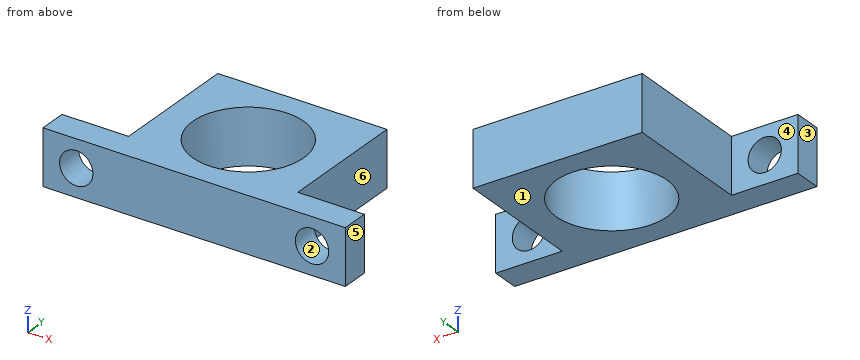
from build123d import *

# Parameters (mm, degrees)
SKETCH_1_R          = 10
EXTRUDE_1_DEPTH     = 10
SKETCH_2_R          = 3
CUT_EXTRUDE_1_DEPTH = 43.114991393


with BuildPart() as part:
    # 草图1 → 凸台-拉伸1 (new body)
    with BuildSketch(Plane.XY):
        Polygon((17.35, 7.3), (-13.15, 7.3), (-13.15, -16.2), (-25.15, -16.2), (-25.15, -21.2), (29.35, -21.2), (29.35, -16.2), (17.35, -16.2), align=None)
        with Locations((2.1, -6.95)):
            Circle(SKETCH_1_R, mode=Mode.SUBTRACT)
    extrude(amount=EXTRUDE_1_DEPTH)

    # 草图2 → 切除-拉伸1 (cut, through all)
    with BuildSketch(Plane(origin=(0, 7.3, 0), x_dir=(1, 0, 0), z_dir=(0, 1, 0))):
        with Locations(Location((-19.15, -5, 0), (0, 0, 180))):
            Circle(SKETCH_2_R)
        with Locations((23.35, -5)):
            Circle(SKETCH_2_R)
    extrude(amount=-CUT_EXTRUDE_1_DEPTH, mode=Mode.SUBTRACT)


solid = part.part
Design review of the part built by this model. Coordinates are the model's own, in mm. Face numbers are marked on the shaded views. A direction names the side the tool comes from. Coordinates: 2 decimals unless noted, no trailing zeros. Order: outer loops, then holes, each group sorted by start corner. A loop starts at its lowest first (then second) coordinate and runs counter-clockwise, first axis right, second up.
Item 1: Take a section at B-B, the plane x = -19.15. Write out the cut boundary in (y, z), then the cut area to 3 significant figures.
Item 2: For line 1 (X direction, y = -17.25, z = 4.75); line 2 (Z direction, x = 23.35, y = -19.7); line 3 (X direction, y = -19.75, z = 7.5), list the stretches that pass through material, from the lowest coordinate up.
Item 3: For pin 1 Ø3 at (y, z) = (-4, 3) entering from -X; pin 2 Ø6 at (y, z) = (-0.5, 3) entering from +X; pin 3 Ø3 at (x, z) = (-18.5, 6.5) entering from +Y, all flat-tipped, find the tip position at first contact; note any pin that passes through.
Item 4: Take a section at C-C, the plane y = -6.95. Write out the cut boundary in (x, z), then the cut area to 3 significant figures.
Item 5: Take a section at D-D, the plane z = 8.5. Write out the cut boundary in (x, y), then the cut area to 3 significant figures.
Item 6: For the marked faces 4, 5 and 6, list the 3-axis set-ups (+Z, -Z, +X, -X, +Y, -Y) from which the entire face can be reached by the end or side of a thin tool; tool diameter is ignored.
Item 7: The part is to be moulded in two halves that separate along X. For the marked faces 1, 2 and 3, say which applies: pulls with the +X half, pulls with the -X half, needs draft (parallel to the pull), parting line crosses it, or undercut.
Item 8: Take a section at A-A, the plane z = 5. Write out the cut boundary in (x, y).
The answers:
1. outline: (-21.2, 0) - (-16.2, 0) - (-16.2, 2) - (-21.2, 2) - close; (-21.2, 8) - (-16.2, 8) - (-16.2, 10) - (-21.2, 10) - close
1. area: 20.0 mm2
2. line 1: x = -25.15 to -22.14, -16.16 to 20.36, 26.34 to 29.35
2. line 2: z = 0 to 2, 8 to 10
2. line 3: x = -25.15 to -20.81, -17.49 to 21.69, 25.01 to 29.35
3. pin 1: stops at x = -13.15
3. pin 2: stops at x = 17.35
3. pin 3: stops at y = -16.2
4. outline: (-13.15, 0) - (-7.9, 0) - (-7.9, 10) - (-13.15, 10) - close; (12.1, 0) - (17.35, 0) - (17.35, 10) - (12.1, 10) - close
4. area: 105 mm2
5. outline: (-25.15, -21.2) - (29.35, -21.2) - (29.35, -16.2) - (17.35, -16.2) - (17.35, 7.3) - (-13.15, 7.3) - (-13.15, -16.2) - (-25.15, -16.2) - close; hole circle Ø20 at (2.1, -6.95)
5. area: 675 mm2
6. face 4: +Z, -Z, -X, +Y
6. face 5: +Z, -Z, +X, +Y, -Y
6. face 6: +Z, -Z, +X, +Y
7. face 1: needs draft
7. face 2: undercut
7. face 3: pulls with the -X half
8. outline: (-25.15, -21.2) - (-22.15, -21.2) - (-22.15, -16.2) - (-25.15, -16.2) - close; (-16.15, -21.2) - (20.35, -21.2) - (20.35, -16.2) - (17.35, -16.2) - (17.35, 7.3) - (-13.15, 7.3) - (-13.15, -16.2) - (-16.15, -16.2) - close; (26.35, -21.2) - (29.35, -21.2) - (29.35, -16.2) - (26.35, -16.2) - close; hole circle Ø20 at (2.1, -6.95)
